from build123d import *

# Parameters (mm, degrees)
F1_DEPTH       = 10
F3_DEPTH       = 10
F5_D           = 4.4
F5_CSINK_D     = 8.96
F5_CSINK_ANGLE = 90
F6_R           = 1
F7_R           = 2
F8_W           = 6
F8_H           = 2.5
F9_DEPTH       = 7.001
F9_DEPTH_BACK  = 20.001
F10_R          = 2


with BuildPart() as f1:
    # F0 (on Front) → F1 (new body)
    with BuildSketch(Plane.XZ):
        Polygon((-13.5, 20.2), (-13.5, 0), (13.5, 0), (13.5, 20.2), (9.5, 20.2), (9.5, 17.2), (11, 17.2), (11, 16), (9.5, 16), (9.5, 3), (-9.5, 3), (-9.5, 16), (-11, 16), (-11, 17.2), (-9.5, 17.2), (-9.5, 20.2), align=None)
    extrude(amount=F1_DEPTH)

    # F2 (on Front) → F3 (join)
    with BuildSketch(Plane.XZ):
        Polygon((-13.5, 0), (13.5, 0), (13.5, 20.2), (6.5, 20.2), (6.5, 6), (-6.5, 6), (-6.5, 20.2), (-13.5, 20.2), align=None)
    extrude(amount=-F3_DEPTH)

    # F5 (through all)
    with Locations(Plane.XY.offset(6)):
        with Locations((0, 5.0612445921)):
            CounterSinkHole(F5_D / 2, F5_CSINK_D / 2, counter_sink_angle=F5_CSINK_ANGLE)

    # F6
    f6_edges = [f1.edges().sort_by_distance(p)[0] for p in [
        (0, -10, 3),
        (-9.5, -10, 9.5),
        (-9.5, -10, 18.7),
        (9.5, -10, 18.7),
        (9.5, -10, 9.5),
    ]]
    fillet(f6_edges, radius=F6_R)

    # F7
    f7_edges = [f1.edges().sort_by_distance(p)[0] for p in [
        (-13.5, 0, 20.2),
        (-13.5, 10, 10.1),
        (13.5, 10, 10.1),
        (13.5, 0, 20.2),
    ]]
    fillet(f7_edges, radius=F7_R)

    # F8 (on face) → F9 (cut, two sides)
    with BuildSketch(Plane.YZ.offset(-6.5)) as f9_sk:
        with Locations((5, 16.95)):
            Rectangle(F8_W, F8_H)
        with Locations((5, 9.25)):
            Rectangle(F8_W, F8_H)
    extrude(amount=-F9_DEPTH, mode=Mode.SUBTRACT)
    extrude(f9_sk.sketch, amount=F9_DEPTH_BACK, mode=Mode.SUBTRACT)

    # F10
    f10_edges = [f1.edges().sort_by_distance(p)[0] for p in [
        (-13.5, 5, 15.7),
        (-13.5, 5, 10.5),
        (13.5, 5, 15.7),
        (13.5, 5, 10.5),
    ]]
    fillet(f10_edges, radius=F10_R)


solid = f1.part
Model file for the job. Use its own axes, mm. A direction names the side the tool comes from. Give positions to 0.01 mm unless a question says otherwise; leave off trailing zeros. Write each loop counter-clockwise with the first axis right and the second up, starting at its lowest first coordinate (ties: lowest second). Pieces come first, ordered by that corner, then holes. Notation, with made-up numbers: (63, -29) -> (95, -29) arc R28 ccw to (95, 6) -> close; hole circle Ø2 at (-38, -35). An arc over 180 degrees is marked (long way). Write item = value, one per line.
(1) Slice it at D-D, the plane x = 8. Give the cut face in (y, z).
Determined:
outline = (-10, 0) -> (10, 0) -> (10, 20.2) -> (0, 20.2) -> (0, 3) -> (-9, 3) arc R1 ccw to (-10, 2) -> close; hole (2, 8) -> (8, 8) -> (8, 10.5) -> (2, 10.5) -> close; hole (2, 15.7) -> (8, 15.7) -> (8, 18.2) -> (2, 18.2) -> close
(2) Tool access for faces 1 (the face through (-11, -5, 17)), 2 (the face through (-9, 5, 15.7)), 3 (the face through (-12.93, 4.96, 11.1)), 4 (the face through (-9.785, -9.699, 9.098)): list every direction of +Z, -Z, +X, -X, +Y, -Y with a clear straight run to the whole face (end or side of a thin tool).
Determined:
face_1 = -Y
face_2 = +X, -X
face_3 = -X
face_4 = +Z, -Y
(3) Slice it at A-A, the plane z = 9. Give the cut face in (x, y), then the cut area to 3 significant figures.
Determined:
outline = (-13.5, -10) -> (-10.5, -10) arc R1 ccw to (-9.5, -9) -> (-9.5, 0) -> (-6.5, 0) -> (-6.5, 2) -> (-13.5, 2) -> close; (-13.5, 8) -> (-6.5, 8) -> (-6.5, 10) -> (-11.5, 10) arc R2 ccw to start; (6.5, 0) -> (9.5, 0) -> (9.5, -9) arc R1 ccw to (10.5, -10) -> (13.5, -10) -> (13.5, 2) -> (6.5, 2) -> close; (6.5, 8) -> (13.5, 8) arc R2 ccw to (11.5, 10) -> (6.5, 10) -> close
area = 134 mm2
(4) Slice it at C-C, the plane y = -5. Give the cut face in (x, z).
Determined:
outline = (-13.5, 0) -> (13.5, 0) -> (13.5, 18.2) arc R2 ccw to (11.5, 20.2) -> (9.5, 20.2) -> (9.5, 17.2) -> (11, 17.2) -> (11, 16) -> (9.5, 16) -> (9.5, 3) -> (-9.5, 3) -> (-9.5, 16) -> (-11, 16) -> (-11, 17.2) -> (-9.5, 17.2) -> (-9.5, 20.2) -> (-11.5, 20.2) arc R2 ccw to (-13.5, 18.2) -> close
(5) Flat gauge pins, fed straight in: P1, Ø3, axis at x = 0.5, y = 6.5, coming from the +Z side; P2, Ø7, axis at x = 0, y = 5.06, coming from the +Z side; P3, Ø4, axis at x = -1.5, y = 0.5, coming from the +Z side. Where does each tip first touch, or does it go through?
Determined:
P1 = 4.54
P2 = 5.02
P3 = 6
(6) Probe line 1 along Z through (x, y) = (6.75, 5.5); line 2 along X through (y, z) = (-8.5, 5.5); line 3 along Y through (x, z) = (0, 1.05). List the from-to ranges inside material, lowest first.
Determined:
line_1 = 0 to 8, 10.5 to 15.7, 18.2 to 20.2
line_2 = -13.5 to -9.5, 9.5 to 13.5
line_3 = -10 to 2.86, 7.26 to 10
(7) Slice it at B-B, the plane x = 0. Give the cut face in (y, z).
Determined:
outline = (-10, 0) -> (2.86, 0) -> (2.86, 3.72) -> (0.58, 6) -> (0, 6) -> (0, 3) -> (-9, 3) arc R1 ccw to (-10, 2) -> close; (7.26, 0) -> (10, 0) -> (10, 6) -> (9.54, 6) -> (7.26, 3.72) -> close
(8) Mould opens along X. For faces 5 (the face through (-12.93, 4.96, 15.1)), 6 (the face through (10, 8, 17)), 7 (the face through (6.5, 5, 13)) say: released by +X, released by -X, zero draft, split by the parting line, or undercut.
Determined:
face_5 = released by -X
face_6 = zero draft
face_7 = undercut
